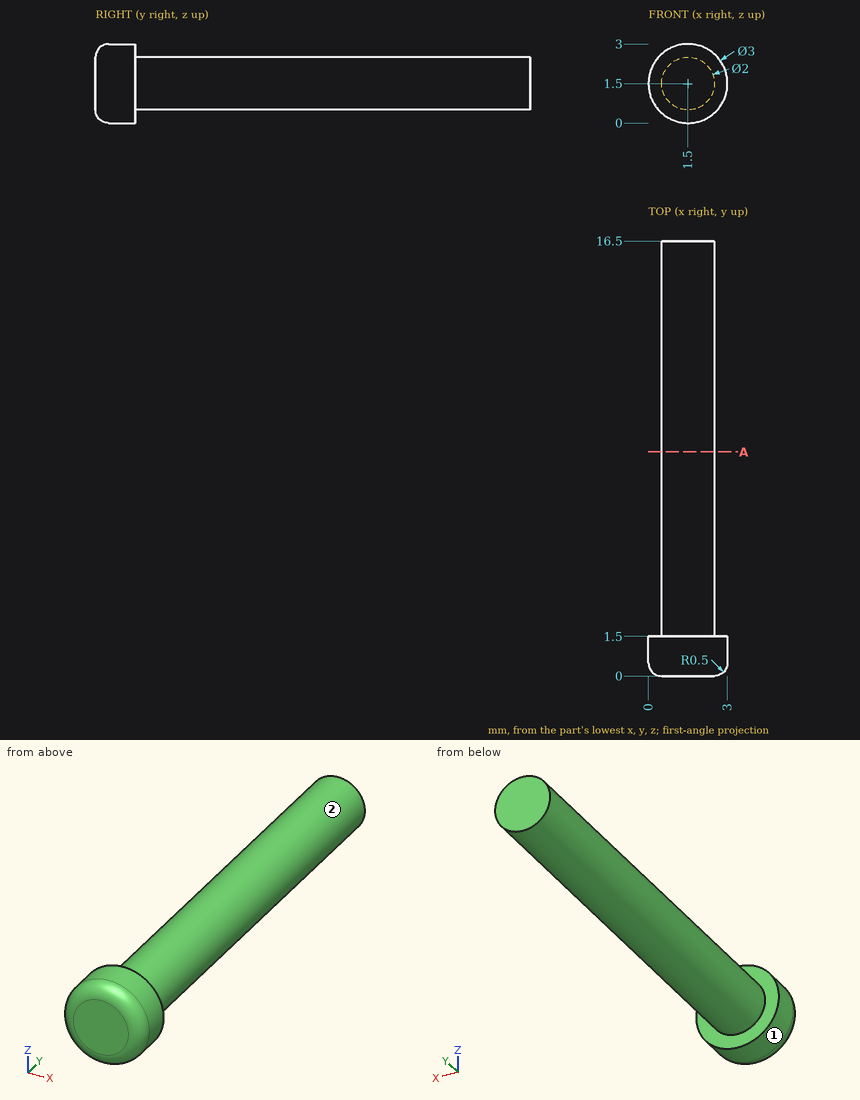
Here's the drawing with two shaded views (mm, measured from the low corner). I have some questions. A direction names the side the tool comes from. Give positions to 0.01 mm unless a question says otherwise; leave off trailing zeros. Write each loop counter-clockwise with the first axis right and the second up, starting at its lowest first coordinate (ties: lowest second). Pieces come first, ordered by that corner, then holes. Notation, with made-up numbers: (11, 39.25) -> (44, 39.25) arc R8 cw to (44, 45.25) -> close; hole circle Ø7 at (-35.5, 50.5). An arc over 180 degrees is marked (long way). Use one line per item in the form item = value.
1) Suppose I cut it at A-A (y = 8.5). Please give me the cut outline in (x, z).
Verdict:
outline = circle Ø2 at (1.5, 1.5)
2) On a 3-axis mill with a long thin cutter (end or side, diameter ignored), from which of +Z, -Z, +X, -X, +Y, -Y can I reach the whole of each face in a straight line? I mean the marked faces 1 and 2. Say none if no direction works.
Verdict:
face_1 = +Y, -Y
face_2 = +Y
3) I'm going to push a flat-ended pin straight in: pin 1 (1.5 mm diameter, centred on x = 1, y = 4, fed in from -Z). Where does the tip first touch, or does it pass through?
Verdict:
pin_1 = 0.5
4) If I drill on L1, parallel to X at y = 15.75, z = 1.45; L2, parallel to Z at x = 2.1, y = 5.5; L3, parallel to X at y = 12.5, z = 0.85, over which ranges is the centre line in solid material (lowest first)? Write a range as [from, to].
Verdict:
L1 = [0.5, 2.5]
L2 = [0.7, 2.3]
L3 = [0.74, 2.26]
